Check sheet for the modelled part. Datum: model origin and axes. Units: mm. Round coordinates to 2 decimals unless told otherwise and drop trailing zeros. Loops run counter-clockwise (first coordinate to the right, second up) from the corner with the lowest first, then second, coordinate; pieces in that order, holes last. Notation, with made-up numbers: (32.25, 25.25) - (65.25, 25.25) arc R32 cw to (65.25, 55.25) - close; hole circle Ø1 at (-18.5, 9). An arc over 180 degrees is marked (long way). Return JSON: item names as keys, results as strings.
from build123d import *

# Parameters (mm, degrees)
EXTRUDE_1_DEPTH          = 1.5
SKETCH_2_W               = 18
SKETCH_2_H               = 18
CUT_EXTRUDE_1_DEPTH      = 3
FILLET_1_R               = 1
FILLET_2_R               = 2
FILLET_3_R               = 3
SKETCH_3_R               = 2.025
CUT_EXTRUDE_2_DEPTH      = 1
CUT_EXTRUDE_2_DEPTH_BACK = 4
SKETCH_4_R               = 2.025
CUT_EXTRUDE_3_DEPTH      = 1
CUT_EXTRUDE_3_DEPTH_BACK = 4
SKETCH_5_R               = 2.025
CUT_EXTRUDE_4_DEPTH      = 1
CUT_EXTRUDE_4_DEPTH_BACK = 4
FILLET_4_R               = 3


with BuildPart() as part:
    # 草图1 → 凸台-拉伸1 (new body, symmetric)
    with BuildSketch(Plane.XY):
        Polygon((40, 0), (-40, 0), (-40, 20), (-15, 90), (15, 90), (40, 20), align=None)
    extrude(amount=EXTRUDE_1_DEPTH, both=True)

    # 草图2 → 切除-拉伸1 (cut)
    with BuildSketch(Plane.XY.offset(1.5)):
        Polygon((-15, 72.160717503), (-33.62882768, 20), (-15, 20), align=None)
        with Locations((0, 64)):
            Rectangle(SKETCH_2_W, SKETCH_2_H)
        with Locations((0, 37)):
            Rectangle(SKETCH_2_W, SKETCH_2_H)
        Polygon((15, 20), (15, 72.160717503), (33.62882768, 20), align=None)
    extrude(amount=-CUT_EXTRUDE_1_DEPTH, mode=Mode.SUBTRACT)

    # 圆角1
    fillet_1_edges = [part.edges().sort_by_distance(p)[0] for p in [
        (-15, 20, 0),
        (-15, 72.160717503, 0),
        (15, 72.160717503, 0),
        (15, 20, 0),
    ]]
    fillet(fillet_1_edges, radius=FILLET_1_R)

    # 圆角2
    fillet_2_edges = [part.edges().sort_by_distance(p)[0] for p in [
        (-9, 46, 0),
        (-9, 28, 0),
        (9, 28, 0),
        (9, 46, 0),
        (-9, 73, 0),
        (-9, 55, 0),
        (9, 55, 0),
        (9, 73, 0),
    ]]
    fillet(fillet_2_edges, radius=FILLET_2_R)

    # 圆角3
    fillet_3_edges = [part.edges().sort_by_distance(p)[0] for p in [
        (40, 0, 0),
        (-40, 0, 0),
        (-40, 20, 0),
        (-15, 90, 0),
        (15, 90, 0),
        (40, 20, 0),
    ]]
    fillet(fillet_3_edges, radius=FILLET_3_R)

    # 草图3 → 切除-拉伸2 (cut, two sides)
    with BuildSketch(Plane.XY.offset(1.5)) as cut_extrude_2_sk:
        with Locations((-27.5, 10)):
            Circle(SKETCH_3_R)
        with Locations((27.5, 10)):
            Circle(SKETCH_3_R)
    extrude(amount=CUT_EXTRUDE_2_DEPTH, mode=Mode.SUBTRACT)
    extrude(cut_extrude_2_sk.sketch, amount=-CUT_EXTRUDE_2_DEPTH_BACK, mode=Mode.SUBTRACT)

    # 草图4 → 切除-拉伸3 (cut, two sides)
    with BuildSketch(Plane.XY.offset(1.5)) as cut_extrude_3_sk:
        with Locations((0, 10)):
            Circle(SKETCH_4_R)
    extrude(amount=CUT_EXTRUDE_3_DEPTH, mode=Mode.SUBTRACT)
    extrude(cut_extrude_3_sk.sketch, amount=-CUT_EXTRUDE_3_DEPTH_BACK, mode=Mode.SUBTRACT)

    # 草图5 → 切除-拉伸4 (cut, two sides)
    with BuildSketch(Plane.XY.offset(1.5)) as cut_extrude_4_sk:
        with Locations((0, 24)):
            Circle(SKETCH_5_R)
        with Locations((0, 50.5)):
            Circle(SKETCH_5_R)
        with Locations((0, 81.5)):
            Circle(SKETCH_5_R)
    extrude(amount=CUT_EXTRUDE_4_DEPTH, mode=Mode.SUBTRACT)
    extrude(cut_extrude_4_sk.sketch, amount=-CUT_EXTRUDE_4_DEPTH_BACK, mode=Mode.SUBTRACT)

    # 圆角4
    fillet_4_edges = [part.edges().sort_by_distance(p)[0] for p in [
        (-33.62882768, 20, 0),
        (33.62882768, 20, 0),
    ]]
    fillet(fillet_4_edges, radius=FILLET_4_R)


solid = part.part
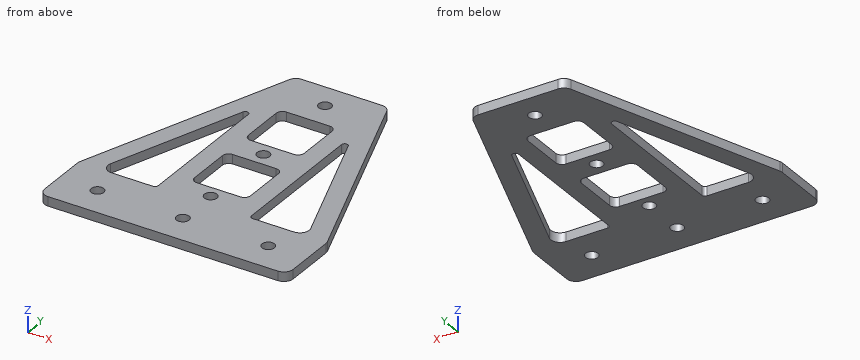
Q1. Depth check by flat-ended pin: P1, Ø1, axis at y = 68, z = 0.5, coming from the +X side; P2, Ø1, axis at y = 48, z = 0.5, coming from the +X side; P3, Ø1, axis at y = 62, z = 1, coming from the +X side; P4, Ø5.5, axis at x = 0, y = 81.5, coming from the +Z side. Enter the tip coordinate at first touch or a pass-through.
Answer key:
{"P1": "stops at x = 23.04", "P2": "stops at x = 30.18", "P3": "stops at x = 25.18", "P4": "stops at z = 1.5"}
Q2. Sectioned sample at C-C (y = 81.5). Enter the section's corners in (x, z) (3 decimals), plus the area to 3 significant figures.
Answer key:
{"outline": "(-18.036, -1.5) - (-2.025, -1.5) - (-2.025, 1.5) - (-18.036, 1.5) - close; (2.025, -1.5) - (18.036, -1.5) - (18.036, 1.5) - (2.025, 1.5) - close", "area": "96.1 mm²"}
Q3. Scan lines: probe 1 along Y at (x, z) = (3, -0.75); probe 2 along X at (y, z) = (39, 0.8); probe 3 along X at (y, z) = (47, 1.3). Record each from-to range of solid material in increasing order. Write a range as [from, to].
Answer key:
{"probe 1": "y = [0, 28], [46, 55], [73, 90]", "probe 2": "x = [-33.21, -26.84], [-15, -9], [9, 15], [26.84, 33.21]", "probe 3": "x = [-30.36, -23.99], [-15, 15], [23.99, 30.36]"}
Q4. Sectioned sample at D-D (z = -0.45). State how many separate pieces and enclosed holes the cut face has, plus the area to 3 significant figures.
Answer key:
{"separate pieces": "1", "enclosed holes": "10", "area": "3,770 mm²"}
Q5. Sectioned sample at B-B (x = 6). Enter the section's corners in (y, z).
Answer key:
{"outline": "(0, -1.5) - (28, -1.5) - (28, 1.5) - (0, 1.5) - close; (46, -1.5) - (55, -1.5) - (55, 1.5) - (46, 1.5) - close; (73, -1.5) - (90, -1.5) - (90, 1.5) - (73, 1.5) - close"}
Q6. Sectioned sample at A-A (y = 10). Enter the section's corners in (x, z) (3 decimals), plus the area to 3 significant figures.
Answer key:
{"outline": "(-40, -1.5) - (-29.525, -1.5) - (-29.525, 1.5) - (-40, 1.5) - close; (-25.475, -1.5) - (-2.025, -1.5) - (-2.025, 1.5) - (-25.475, 1.5) - close; (2.025, -1.5) - (25.475, -1.5) - (25.475, 1.5) - (2.025, 1.5) - close; (29.525, -1.5) - (40, -1.5) - (40, 1.5) - (29.525, 1.5) - close", "area": "204 mm²"}
